Source: CAD feature listing. Evaluate the final solid. Frame: model axes, mm. A direction names the side the tool comes from. Give positions to 0.01 mm unless a question says otherwise; leave off trailing zeros. Order: outer loops, then holes, each group sorted by start corner. A loop starts at its lowest first (then second) coordinate and runs counter-clockwise, first axis right, second up. Notation, with made-up numbers: (-17.5, -38) - (26.5, -38) arc R25 ccw to (26.5, -9) - close; hole circle Ø5 at (41.25, -8). An arc over 180 degrees is marked (long way). Answer as CSV lines item,"result".
```python
from build123d import *

# Parameters (mm, degrees)
SKETCH_1_R          = 3.5
EXTRUDE_1_DEPTH     = 3.9
EXTRUDE_START       = 2.4
SKETCH_1_6_R        = 0.6
EXTRUDE_2_DEPTH     = 1.5
SKETCH_1_3_R        = 2.5
CUT_EXTRUDE_1_DEPTH = 2
CUT_EXTRUDE_START   = 3.9
SKETCH_1_4_R        = 1.5
CUT_EXTRUDE_2_DEPTH = 1
SKETCH_1_5_R        = 1
CUT_EXTRUDE_3_DEPTH = 17.788761122


with BuildPart() as part:
    # 草图1 → 凸台-拉伸1 (new body)
    with BuildSketch(Plane.XY):
        Circle(SKETCH_1_R)
    extrude(amount=EXTRUDE_1_DEPTH)

    # 草图1<6> → 凸台-拉伸2 (add)
    with BuildSketch(Plane.XY.offset(EXTRUDE_START)):
        with BuildLine():
            Line((14.170277633, 1.89618915), (2.286372673, 2.65))
            ThreePointArc((2.286372673, 2.65), (3.5, 0), (2.286372673, -2.65))
            Line((2.286372673, -2.65), (14.170277633, -1.89618915))
            ThreePointArc((14.170277633, -1.89618915), (15.95, 0), (14.170277633, 1.89618915))
        make_face()
        with BuildLine():
            ThreePointArc((11.54, 0), (12.14, 0.6), (12.74, 0))
            ThreePointArc((12.74, 0), (12.14, -0.6), (11.54, 0))
        make_face(mode=Mode.SUBTRACT)
        with Locations((4.5, 0)):
            Circle(SKETCH_1_6_R, mode=Mode.SUBTRACT)
        with BuildLine():
            ThreePointArc((5.81, 0), (6.41, 0.6), (7.01, 0))
            ThreePointArc((7.01, 0), (6.41, -0.6), (5.81, 0))
        make_face(mode=Mode.SUBTRACT)
        with BuildLine():
            ThreePointArc((7.72, 0), (8.32, 0.6), (8.92, 0))
            ThreePointArc((8.92, 0), (8.32, -0.6), (7.72, 0))
        make_face(mode=Mode.SUBTRACT)
        with BuildLine():
            ThreePointArc((9.63, 0), (10.23, 0.6), (10.83, 0))
            ThreePointArc((10.83, 0), (10.23, -0.6), (9.63, 0))
        make_face(mode=Mode.SUBTRACT)
        with Locations((14.05, 0)):
            Circle(SKETCH_1_6_R, mode=Mode.SUBTRACT)
    extrude_2 = extrude(amount=EXTRUDE_2_DEPTH)

    # 镜向1: 凸台-拉伸2 across plane
    add(extrude_2.mirror(Plane(origin=(0, 0, 0), x_dir=(0, 0, 1), z_dir=(1, 0, 0))))

    # 草图1<3> → 切除-拉伸1 (cut)
    with BuildSketch(Plane.XY):
        Circle(SKETCH_1_3_R)
    extrude(amount=CUT_EXTRUDE_1_DEPTH, mode=Mode.SUBTRACT)

    # 草图1<4> → 切除-拉伸2 (cut)
    with BuildSketch(Plane.XY.offset(CUT_EXTRUDE_START)):
        Circle(SKETCH_1_4_R)
    extrude(amount=-CUT_EXTRUDE_2_DEPTH, mode=Mode.SUBTRACT)

    # 草图1<5> → 切除-拉伸3 (cut, through all)
    with BuildSketch(Plane.XY):
        Circle(SKETCH_1_5_R)
    extrude(amount=CUT_EXTRUDE_3_DEPTH, mode=Mode.SUBTRACT)


solid = part.part
```
(1) Cut plane A-A (z = 3.55). Give the number of separate pieces and of enclosed holes in the cut face, then the cut area to 3 significant figures.
Completed:
separate pieces,"1"
enclosed holes,"13"
area,"127 mm²"
(2) Access query for faces 1 (the cylindrical face through (3.233, -1.341, 1.489)), 2 (the cylindrical face through (-8.874, 0.23, 3.14)). Directions: +Z, -Z, +X, -X, +Y, -Y. A direction counts if a zero-diameter tool reaches every point of the face in a straight line with its end or side. Return the directions, or none.
Completed:
face 1,"-Z"
face 2,"+Z, -Z"
(3) Cut plane B-B (x = 0). Return loops of the section in (y, z).
Completed:
outline,"(-3.5, 0) - (-2.5, 0) - (-2.5, 2) - (-1, 2) - (-1, 2.9) - (-1.5, 2.9) - (-1.5, 3.9) - (-3.5, 3.9) - close; (1, 2) - (2.5, 2) - (2.5, 0) - (3.5, 0) - (3.5, 3.9) - (1.5, 3.9) - (1.5, 2.9) - (1, 2.9) - close"
(4) Cut plane D-D (x = -8). Return loops of the section in (y, z).
Completed:
outline,"(-2.29, 2.4) - (-0.51, 2.4) - (-0.51, 3.9) - (-2.29, 3.9) - close; (0.51, 2.4) - (2.29, 2.4) - (2.29, 3.9) - (0.51, 3.9) - close"
(5) Contact query for flat-ended pins moving along their axis: pin 1 (1.4 mm diameter, centred on x = 6.41, y = 0, fed in from -Z); pin 2 (2.5 mm diameter, centred on x = 0, y = 0, fed in from -Z). Output: stop coordinate, or through.
Completed:
pin 1,"z = 2.4"
pin 2,"z = 2"
(6) Mould query, pull axis Y, two halves, no side actions, for faces 3 (the cylindrical face through (-6.28, 0.586, 3.14)), 4 (the flat face through (8.312, 2.268, 3.14)), 5 (the cylindrical face through (-15.95, -0.04, 3.14)). Classes: released by +Y, released by -Y, zero draft, split by the parting line, or undercut.
Completed:
face 3,"undercut"
face 4,"released by +Y"
face 5,"split by the parting line"
(7) Ray query, line 1 (Y direction, x = 0, z = 2.35); line 2 (Y direction, x = 1, z = 1.45); line 3 (Z direction, x = 13.5, y = -1.25). Return the intervals inside material, ascending. Write a range as from..to.
Completed:
line 1,"-3.5..-1, 1..3.5"
line 2,"-3.35..-2.29, 2.29..3.35"
line 3,"2.4..3.9"
(8) Cut plane C-C (z = 0.55). Return loops of the section in (x, y).
Completed:
outline,"circle Ø7 at (0, 0); hole circle Ø5 at (0, 0)"
